from build123d import *

# Parameters (mm, degrees)
F1_DEPTH = 13
F2_W     = 110
F2_H     = 15
F3_DEPTH = 25
F4_R     = 7.5
F5_DEPTH = 25


with BuildPart() as f1:
    # F0 (on Front) → F1 (new body)
    with BuildSketch(Plane.XZ):
        with BuildLine():
            Line((136.328066, 118.956802), (-120.671934, 118.956802))
            ThreePointArc((-120.671934, 118.956802), (-134.814069, 113.098938), (-140.671934, 98.956802))
            Line((-140.671934, 98.956802), (-140.671934, -91.043198))
            Line((-140.671934, -91.043198), (156.328066, -91.043198))
            Line((156.328066, -91.043198), (156.328066, 98.956802))
            ThreePointArc((156.328066, 98.956802), (150.470202, 113.098938), (136.328066, 118.956802))
        make_face()
    extrude(amount=F1_DEPTH)

    # F2 (on face) → F3 (cut)
    with BuildSketch(Plane.XZ.offset(13)):
        with Locations((105.148206, 72.65589)):
            Rectangle(F2_W, F2_H)
    extrude(amount=-F3_DEPTH, mode=Mode.SUBTRACT)

    # F4 (on face) → F5 (join)
    with BuildSketch(Plane.XZ.offset(13)):
        with Locations((-116.048563, 98.956802)):
            Circle(F4_R)
        with Locations((-91.048563, 98.956802)):
            Circle(F4_R)
    extrude(amount=F5_DEPTH)


solid = f1.part
The model under review builds one solid part; all positions refer to its coordinate system, in mm. A direction names the side the tool comes from. Round coordinates to 2 decimals unless told otherwise and drop trailing zeros. Order: outer loops, then holes, each group sorted by start corner. A loop starts at its lowest first (then second) coordinate and runs counter-clockwise, first axis right, second up. Notation, with made-up numbers: (15.5, 72.25) -> (53.5, 72.25) arc R28 ccw to (53.5, 90.25) -> close; hole circle Ø4 at (21.25, -14.5). An arc over 180 degrees is marked (long way). Write item = value, one per line. Start each with the question number.
Item 1: Clearance check with flat-ended pins moving along their axes: pin 1 Ø5 at (x, y) = (-59, -17) entering from +Z; pin 2 Ø10.5 at (y, z) = (-3.5, 73.5) entering from +X; pin 3 Ø5 at (x, z) = (98.5, -23) entering from -Y. State where each tip first meets the part, or that it passes through.
Item 2: Consider section A-A on x = 130. Write out the cut boundary in (y, z), plus the area to 4 significant figures.
Item 3: Mouldability with a two-part tool opening along Z and no side actions: class faces 1 (the face through (156.328, -6, -14)), 2 (the face through (102, -7, 80.156)), 3 (the face through (150.625, -6.409, 112.943)) as released by +Z, released by -Z, zero draft, split by the parting line, or undercut.
Item 4: For faces 4 (the face through (-140.672, -6, 5)), 5 (the face through (50.148, -7, 73)), 6 (the face through (-98.54, -25.32, 99.29)), list the 3-axis set-ups (+Z, -Z, +X, -X, +Y, -Y) from which the entire face can be reached by the end or side of a thin tool; tool diameter is ignored.
Item 5: Consider section D-D on z = 49. Write out the cut boundary in (x, y), plus the area to 3 significant figures.
Item 6: Consider section C-C on y = -34. Write out the cut boundary in (x, z), plus the area to 3 significant figures.
Item 7: For line 1 along Y through (x, z) = (-121.5, 8); line 2 along X through (y, z) = (-34, 103.5); line 3 along X through (y, z) = (-26.5, 96), list the stretches that pass through material, from the lowest coordinate up.
Item 8: Consider section B-B on y = -6.5. Write out the cut boundary in (x, z), plus the area to 3 significant figures.
Conclusion:
q1.pin_1 = through
q1.pin_2 = 50.15
q1.pin_3 = -13
q2.outline = (-13, -91.04) -> (0, -91.04) -> (0, 65.16) -> (-13, 65.16) -> close; (-13, 80.16) -> (0, 80.16) -> (0, 118.96) -> (-13, 118.96) -> close
q2.area = 2,535 mm2
q3.face_1 = zero draft
q3.face_2 = undercut
q3.face_3 = released by +Z
q4.face_4 = +Z, -Z, -X, +Y, -Y
q4.face_5 = +X, +Y, -Y
q4.face_6 = -Y
q5.outline = (-140.67, -13) -> (156.33, -13) -> (156.33, 0) -> (-140.67, 0) -> close
q5.area = 3,860 mm2
q6.outline = circle Ø15 at (-116.05, 98.96); circle Ø15 at (-91.05, 98.96)
q6.area = 353 mm2
q7.line_1 = -13 to 0
q7.line_2 = -122.02 to -110.08, -97.02 to -85.08
q7.line_3 = -122.94 to -109.16, -97.94 to -84.16
q8.outline = (-140.67, -91.04) -> (156.33, -91.04) -> (156.33, 65.16) -> (50.15, 65.16) -> (50.15, 80.16) -> (156.33, 80.16) -> (156.33, 98.96) arc R20 ccw to (136.33, 118.96) -> (-120.67, 118.96) arc R20 ccw to (-140.67, 98.96) -> close
q8.area = 60,600 mm2
